CAD build for the part. Positions are in the model's coordinates, mm. A direction names the side the tool comes from. Coordinates: 2 decimals unless noted, no trailing zeros. Loops run counter-clockwise (first coordinate to the right, second up) from the corner with the lowest first, then second, coordinate; pieces in that order, holes last. Notation, with made-up numbers: (-25, 50.5) -> (24, 50.5) arc R29 ccw to (24, 70.5) -> close; hole circle Ø8 at (87, 19.5). An arc over 180 degrees is marked (long way). Return JSON: item names as keys, results as strings. Group by question number.
(1) Tool access for faces 1 (the face through (43.555, 185, 19)), 2 (the face through (48, 185, 15.24)), 3 (the face through (34, 150, 15.24)): list every direction of +Z, -Z, +X, -X, +Y, -Y with a clear straight run to the whole face (end or side of a thin tool).
(2) Flat gauge pins, fed straight in: pin 1 Ø3 at (x, y) = (32, 156.5) entering from +Z; pin 2 Ø1.5 at (y, z) = (182, 4.5) entering from +X; pin 3 Ø7 at (x, z) = (30.5, 7.5) entering from +Y; pin 4 Ø6 at (y, z) = (185.5, 20) entering from -X. Where does each tip first touch, or does it go through?
(3) Probe L1, parallel to Z at x = 34, y = 151; L2, parallel to Y at x = 29, z = 13.5; L3, parallel to X at y = 180.5, z = 16. List the from-to ranges inside material, lowest first.
(4) Saw through at D-D on x = 29. Write the cut outline in (y, z), then the cut area to 3 significant figures.
(5) Saw through at C-C on z = 2.75. Write the cut outline in (x, y).
(6) Saw through at A-A on x = 45.5. Write the cut outline in (y, z), then the cut area to 3 significant figures.
(7) Saw through at B-B on y = 172. Write the cut outline in (x, z), then the cut area to 3 significant figures.
Autodesk Inventor part; units mm, degrees
ref_plane "YZ Plane" through (0, 0, 0) normal (1, 0, 0) x (0, 1, 0)
ref_plane "XZ Plane" through (0, 0, 0) normal (0, 1, 0) x (-1, 0, 0)
ref_plane "XY Plane" through (0, 0, 0) normal (0, 0, 1) x (1, 0, 0)
sketch "Sketch1" plane through (0, 0, 0) normal (0, 0, 1) x (1, 0, 0)
  line L0 (52.1911, 179.7031) -> (21.9651, 179.7031)
  line L1 (21.9651, 179.7031) -> (21.9651, 130.4271)
  line L2 (21.9651, 130.4271) -> (52.1911, 130.4271)
  line L3 (52.1911, 130.4271) -> (52.1911, 179.7031)
  point P0 (0, 0)
  dimension "d0" = 30.226
  dimension "d1" = 49.276
extrude "Extrusion1" add sketch "Sketch1" along normal blind 15.24
sketch "Sketch2" plane through (0, 0, 15.24) normal (0, 0, 1) x (1, 0, 0)
  line L0 (52.1911, 179.7031) -> (52.1911, 130.4271)
  line L1 (21.9651, 179.7031) -> (52.1911, 179.7031)
  line L2 (52.1911, 171.0671) -> (43.5551, 171.0671)
  line L3 (43.5551, 171.0671) -> (43.5551, 190.3711)
  line L4 (43.5551, 190.3711) -> (52.1911, 190.3711)
  line L5 (52.1911, 190.3711) -> (52.1911, 171.0671)
  point P0 (0, 0)
  dimension "d4" = 8.636
  dimension "d5" = 8.636
  dimension "d6" = 10.668
extrude "Extrusion2" add sketch "Sketch2" along normal blind 7.366
fillet "Fillet1" radius 12.7 2 edges at (43.5551, 175.3851, 15.24) (47.8731, 171.0671, 15.24)
properties part number "Rangelink Reciever"
Geometry results:
{
 "1": {"face 1": "+Z, -Z, -X, +Y", "face 2": "-Z, +X, -X, +Y", "face 3": "+Z, -X, -Y"},
 "2": {"pin 1": "z = 15.24", "pin 2": "through", "pin 3": "y = 179.7", "pin 4": "x = 43.56"},
 "3": {"L1": "0 to 15.24", "L2": "130.43 to 179.7", "L3": "43.56 to 52.19"},
 "4": {"outline": "(130.43, 0) -> (179.7, 0) -> (179.7, 15.24) -> (130.43, 15.24) -> close", "area": "751 mm²"},
 "5": {"outline": "(21.97, 130.43) -> (52.19, 130.43) -> (52.19, 179.7) -> (21.97, 179.7) -> close"},
 "6": {"outline": "(130.43, 0) -> (179.7, 0) -> (179.7, 15.24) -> (190.37, 15.24) -> (190.37, 22.61) -> (171.07, 22.61) arc R12.7 cw to (159.54, 15.24) -> (130.43, 15.24) -> close", "area": "917 mm²"},
 "7": {"outline": "(21.97, 0) -> (52.19, 0) -> (52.19, 22.61) -> (43.56, 22.61) arc R12.7 cw to (32.03, 15.24) -> (21.97, 15.24) -> close", "area": "548 mm²"}
}
